from build123d import *

# Parameters (mm, degrees)
BOSS_EXTRUDE1_DEPTH = 10


with BuildPart() as part:
    # Sketch1 → Boss-Extrude1 (new body)
    with BuildSketch(Plane(origin=(0, 0, 0), x_dir=(1, 0, 0), z_dir=(0, 1, 0))):
        with BuildLine():
            ThreePointArc((14.028659191, 32.065506722), (-35, 0), (14.028659191, -32.065506722))
            Line((14.028659191, -32.065506722), (50.674952587, -16.032753361))
            ThreePointArc((50.674952587, -16.032753361), (61.160622991, 0), (50.674952587, 16.032753361))
            Line((50.674952587, 16.032753361), (14.028659191, 32.065506722))
        make_face()
        with BuildLine():
            Line((9.886859967, 1.5), (14.886859967, 1.5))
            Line((14.886859967, 1.5), (14.886859967, -1.5))
            Line((14.886859967, -1.5), (9.886859967, -1.5))
            ThreePointArc((9.886859967, -1.5), (-10, 0), (9.886859967, 1.5))
        make_face(mode=Mode.SUBTRACT)
    extrude(amount=BOSS_EXTRUDE1_DEPTH)


solid = part.part
Can you work these out from the model? Positions are in its coordinate system, mm. A direction names the side the tool comes from. Give positions to 0.01 mm unless a question says otherwise; leave off trailing zeros. Order: outer loops, then holes, each group sorted by start corner. A loop starts at its lowest first (then second) coordinate and runs counter-clockwise, first axis right, second up. Notation, with made-up numbers: M -6,52 L 19,52 A14 cw 19,70 Z; hole C -23,22 d10. An arc over 180 degrees is marked long. Use one line per item in the form item = value.
Item 1: If we section it at B-B, the plane x = 0: Write out the boundary of the cut face in (y, z).
Values follow:
outline = M 0,-35 L 10,-35 L 10,-10 L 0,-10 Z; M 0,10 L 10,10 L 10,35 L 0,35 Z
Item 2: Will these pins go through, and if not, where does the flat tip stop? pin 1 Ø4 at (x, y) = (12.5, 5) entering from -Z; pin 2 Ø3.5 at (y, z) = (4, 0.5) entering from -X; pin 3 Ø10 at (x, z) = (48.5, -24) entering from +Y; pin 4 Ø3 at (x, z) = (-7.5, 8.5) entering from -Y.
Values follow:
pin_1 = -33.39
pin_2 = -35
pin_3 = through
pin_4 = 0
Item 3: If we section it at D-D, the plane z = -23: Write out the boundary of the cut face in (x, y).
Values follow:
outline = M -26.38,0 L 34.75,0 L 34.75,10 L -26.38,10 Z
Item 4: If we section it at A-A, the plane z = 0: Write out the boundary of the cut face in (x, y), and give its area (3 significant figures).
Values follow:
outline = M -35,0 L -10,0 L -10,10 L -35,10 Z; M 14.89,0 L 61.16,0 L 61.16,10 L 14.89,10 Z
area = 713 mm^2
Item 5: Thinking about a two-plate mould opening in Z: for faces 1 (the flat face through (14.887, 5, 0)), 2 (the flat face through (32.1, 4.93, 24.16)), 3 (the cylindrical face through (-34.987, 4.93, -0.972)), which applies, pulls with the +Z half, pulls with the -Z half, needs draft (parallel to the pull), parting line crosses it, or undercut?
Values follow:
face_1 = undercut
face_2 = pulls with the +Z half
face_3 = parting line crosses it
Item 6: If we section it at C-C, the plane y = 8: Write out the boundary of the cut face in (x, z), and give its area (3 significant figures).
Values follow:
outline = M 14.03,-32.07 L 50.67,-16.03 A17.5 ccw 50.67,16.03 L 14.03,32.07 A35 ccw long Z; hole M 9.89,-1.5 L 14.89,-1.5 L 14.89,1.5 L 9.89,1.5 A10 ccw long Z
area = 4,560 mm^2
Item 7: For faces 4 (the flat face through (32.608, 4.93, -23.937)), 5 (the flat face through (12, 5, -1.5)), which set-ups out of +Z, -Z, +X, -X, +Y, -Y let a thin tool reach every point of the face, with its end or its side?
Values follow:
face_4 = -Z, +X, +Y, -Y
face_5 = +Y, -Y
Item 8: If I drill on line 1 along Z through (x, y) = (0, 5.25); line 2 along X through (y, z) = (2.25, 3); line 3 along X through (y, z) = (1.25, 3.5), over which ranges is the centre line in solid material (lowest first)? Write a range as [from, to].
Values follow:
line_1 = [-35, -10], [10, 35]
line_2 = [-34.87, -9.54], [9.54, 60.9]
line_3 = [-34.82, -9.37], [9.37, 60.81]
